```python
from build123d import *

# Parameters (mm, degrees)
SKETCH1_W           = 80
SKETCH1_H           = 60
BOSS_EXTRUDE1_DEPTH = 21
CUT_EXTRUDE1_DEPTH  = 21
SKETCH3_W           = 70
SKETCH3_H           = 55
CUT_EXTRUDE2_DEPTH  = 17


with BuildPart() as part:
    # Sketch1 → Boss-Extrude1 (new body)
    with BuildSketch(Plane(origin=(0, 0, 0), x_dir=(0, 0, -1), z_dir=(1, 0, 0))):
        Rectangle(SKETCH1_W, SKETCH1_H)
    extrude(amount=BOSS_EXTRUDE1_DEPTH)

    # Sketch2 → Cut-Extrude1 (cut)
    with BuildSketch(Plane(origin=(21, 0, 0), x_dir=(0, 0, -1), z_dir=(1, 0, 0))):
        with BuildLine():
            ThreePointArc((7.79, 11.5), (-16.21, -12.5), (7.79, -36.5))
            ThreePointArc((7.79, -36.5), (11.79, -32.5), (7.79, -28.5))
            ThreePointArc((7.79, -28.5), (-8.21, -12.5), (7.79, 3.5))
            ThreePointArc((7.79, 3.5), (11.79, 7.5), (7.79, 11.5))
        make_face()
    extrude(amount=-CUT_EXTRUDE1_DEPTH, mode=Mode.SUBTRACT)

    # Sketch3 → Cut-Extrude2 (cut)
    with BuildSketch(Plane.ZY):
        with Locations((0, -2.5)):
            Rectangle(SKETCH3_W, SKETCH3_H)
    extrude(amount=-CUT_EXTRUDE2_DEPTH, mode=Mode.SUBTRACT)


solid = part.part
```
Can you work these out from the model? Positions are in its coordinate system, mm. A direction names the side the tool comes from. Give positions to 0.01 mm unless a question says otherwise; leave off trailing zeros. Order: outer loops, then holes, each group sorted by start corner. A loop starts at its lowest first (then second) coordinate and runs counter-clockwise, first axis right, second up. Notation, with made-up numbers: (30.5, 43.5) - (78.5, 43.5) arc R21 ccw to (78.5, 75.5) - close; hole circle Ø9 at (11, 35.25). An arc over 180 degrees is marked (long way). Use a Markdown table: item, result. Add a question column.
Q1. On a 3-axis mill with a long thin cutter (end or side, diameter ignored), from which of +Z, -Z, +X, -X, +Y, -Y can I reach the whole of each face in a straight line? I mean faces 1 (the cylindrical face through (19.03, 7.41, -11.79)), 2 (the cylindrical face through (19.028, -28.905, -9.545)), 3 (the flat face through (8, -3, 35)), 4 (the flat face through (21, 0, 1)), 5 (the flat face through (17.5, -30, 30.2)). Say none if no direction works.
Q2. If we section it at B-B on y = 18.5: Write out the boundary of the cut face in (x, z).
Q3. If we section it at A-A on y = -12.5: Write out the boundary of the cut face in (x, z), plus the area to 3 significant figures.
Q4. If we mould it in two halves opening along Y, with no side actions, what happens to faces 6 (the flat face through (17.5, -30, -28.6)), 7 (the flat face through (0, 27, 6)), 8 (the cylindrical face through (19.028, -3.296, 14.375)), 9 (the cylindrical face through (19.028, -12.852, 8.206))? For each: released by +Y, released by -Y, zero draft, split by the parting line, or undercut.
Q5. I'm going to push a flat-ended pin straight in: pin 1 (12 mm diameter, centred on y = 11, z = 0, fed in from -X). Where does the tip first touch, or does it pass through?
Q6. If we section it at D-D on x = 7: Write out the boundary of the cut face in (y, z).
Q7. If we section it at C-C on z = -1.5: Write out the boundary of the cut face in (x, y).
Q8. Please list where these lines run through material, in increasing order: line 1 along Z through (x, y) = (3.5, 21); line 2 along Z through (x, y) = (17.5, 5); line 3 along Y through (x, z) = (3, 21).
Answers follow:
| question | item | result |
|---|---|---|
| 1 | face 1 | +X, -X |
| 1 | face 2 | +X, -X, -Y |
| 1 | face 3 | -X, -Y |
| 1 | face 4 | +Z, -Z, +X, +Y, -Y |
| 1 | face 5 | +Z, -Z, +X, -X, -Y |
| 2 | outline | (0, -40) - (21, -40) - (21, 40) - (0, 40) - (0, 35) - (17, 35) - (17, -35) - (0, -35) - close |
| 3 | outline | (0, -40) - (21, -40) - (21, 8.21) - (17, 8.21) - (17, -35) - (0, -35) - close; (0, 35) - (17, 35) - (17, 16.21) - (21, 16.21) - (21, 40) - (0, 40) - close |
| 3 | area | 458 mm^2 |
| 4 | face 6 | released by -Y |
| 4 | face 7 | zero draft |
| 4 | face 8 | undercut |
| 4 | face 9 | undercut |
| 5 | pin 1 | stops at x = 17 |
| 6 | outline | (-30, -40) - (30, -40) - (30, 40) - (-30, 40) - (-30, 35) - (25, 35) - (25, -35) - (-30, -35) - close |
| 7 | outline | (0, 25) - (17, 25) - (17, 10.66) - (21, 10.66) - (21, 30) - (0, 30) - close; (17, -27.21) - (21, -27.21) - (21, 2.21) - (17, 2.21) - close |
| 8 | line 1 | z = -40 to -35, 35 to 40 |
| 8 | line 2 | z = -40 to -10.91, 8.63 to 40 |
| 8 | line 3 | y = 25 to 30 |
